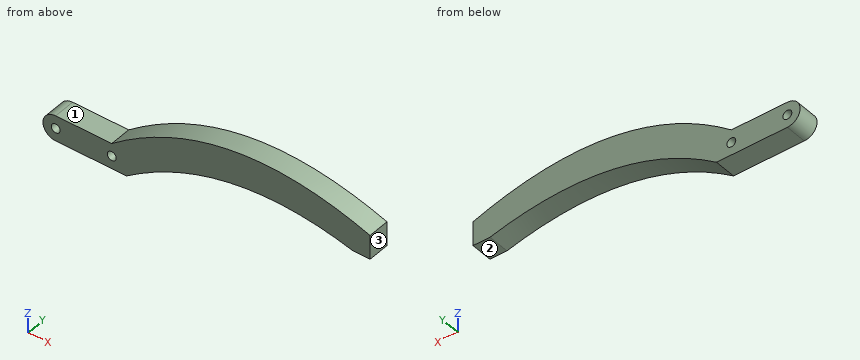
from build123d import *

# Parameters (mm, degrees)
CROQUIS2_R              = 1.75
SALIENTE_EXTRUIR1_DEPTH = 8.5


with BuildPart() as part:
    # Croquis2 → Saliente-Extruir1 (new body)
    with BuildSketch(Plane(origin=(0, 0, 0), x_dir=(1, 0, 0), z_dir=(0, 1, 0))):
        with BuildLine():
            Line((-22, -5), (0, -5))
            add(Edge.make_bspline(
                [(0, -5), (44.060717463, -39.575226666), (101.432631882, -19.199942723)],
                knots=[0, 0, 0, 1, 1, 1], degree=2))
            Line((101.432631882, -19.199942723), (101.432631882, -9.706723131))
            Line((101.432631882, -9.706723131), (94.748347294, -9.706723131))
            add(Edge.make_bspline(
                [(5.809010248, 5), (44.703591594, -23.148227448), (94.748347294, -9.706723131)],
                knots=[0, 0, 0, 1, 1, 1], degree=2))
            Line((5.809010248, 5), (0, 5))
            Line((0, 5), (-0.763110027, 5))
            Line((-0.763110027, 5), (-22, 5))
            ThreePointArc((-22, 5), (-27, 0), (-22, -5))
        make_face()
        with Locations(Location((-22, 0, 0), (0, 0, 270))):
            Circle(CROQUIS2_R, mode=Mode.SUBTRACT)
        with Locations(Location((0, 0, 0), (0, 0, 270))):
            Circle(CROQUIS2_R, mode=Mode.SUBTRACT)
    extrude(amount=SALIENTE_EXTRUIR1_DEPTH)


solid = part.part
Verification items for the finished model (mm, model axes). Face numbers are marked on the shaded views. A direction names the side the tool comes from. Coordinates: 2 decimals unless noted, no trailing zeros. Write each loop counter-clockwise with the first axis right and the second up, starting at its lowest first coordinate (ties: lowest second). Pieces come first, ordered by that corner, then holes. Notation, with made-up numbers: (15, -18.5) - (37, -18.5) arc R20 cw to (37, -13.5) - close; hole circle Ø2 at (-33.5, 21). An arc over 180 degrees is marked (long way). Answer as a JSON object with one key per item and string values.
(1) Cross-section at B-B on x = -5. Record the cut outline in (y, z), plus the area to 3 significant figures.
Report:
{"outline": "(0, -5) - (8.5, -5) - (8.5, 5) - (0, 5) - close", "area": "85.0 mm^2"}
(2) Thickness scan on line 1 along X through (y, z) = (6, 0); line 2 along X through (y, z) = (5.5, -1.5); line 3 along Z through (x, y) = (-19, 1.5). Record the ranges inside material, lowest first.
Report:
{"line 1": "-27 to -23.75, -20.25 to -1.75, 1.75 to 13.34", "line 2": "-26.77 to -22.9, -21.1 to -0.9, 0.9 to 10.94", "line 3": "-5 to 5"}
(3) Gauge pin test, flat ends, axial feed: pin 1 Ø2 at (x, y) = (65, 2) entering from +Z; pin 2 Ø1 at (x, y) = (55, 4.5) entering from +Z; pin 3 Ø4 at (x, y) = (-6.5, 5.5) entering from +Z. Record the tip position at first contact, or that the pin passes through.
Report:
{"pin 1": "z = 26.7", "pin 2": "z = 26.62", "pin 3": "z = 5"}
(4) Cross-section at A-A on y = 5. Give the number of separate pieces and of enclosed holes in the cut face, plus the area to 3 significant figures.
Report:
{"separate pieces": "1", "enclosed holes": "2", "area": "1,540 mm^2"}
(5) Tool access check on the marked faces 1, 2 and 3. Record the directions out of +Z, -Z, +X, -X, +Y, -Y that give a thin tool (end or side, any length) a straight path to the whole face; none if there is none.
Report:
{"face 1": "+Z, -X, +Y, -Y", "face 2": "-Z, +X, +Y, -Y", "face 3": "+Z, -Z, +X, +Y, -Y"}
